Can you work these out from the drawing? Everything is in mm from the part's minimum corner. Round coordinates to 2 decimals unless told otherwise and drop trailing zeros. Loops run counter-clockwise (first coordinate to the right, second up) from the corner with the lowest first, then second, coordinate; pieces in that order, holes last. Notation, with made-up numbers: M -37.75,21.5 L 21.25,21.5 A18 cw 21.25,41.5 Z; hole C 75,23.5 d7. An arc over 180 degrees is marked long. Use a Markdown table: item, result.
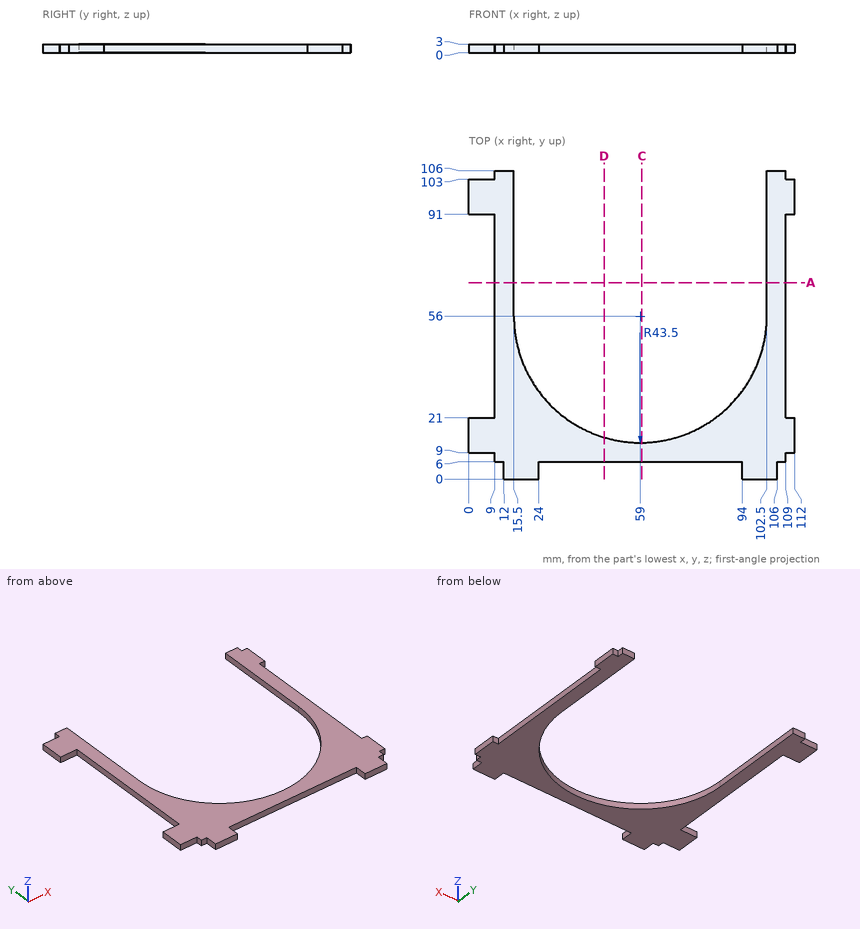
1. Imagine slicing it at D-D, the plane x = 46.5. Write out the boundary of the cut face in (y, z).
Answer sheet:
| item | result |
|---|---|
| outline | M 6,0 L 14.33,0 L 14.33,3 L 6,3 Z |
2. Imagine slicing it at C-C, the plane x = 59.5. Write out the boundary of the cut face in (y, z).
Answer sheet:
| item | result |
|---|---|
| outline | M 6,0 L 12.5,0 L 12.5,3 L 6,3 Z |
3. I need wall thicknesses on probe 1 along X at (y, z) = (63.5, 2.6); probe 2 along Y at (x, z) = (5, 1.8); probe 3 along X at (y, z) = (5.5, 0.25). Which ranges of each line are inside material? Lowest first, please. Write a range as from..to.
Answer sheet:
| item | result |
|---|---|
| probe 1 | 9..15.5, 102.5..109 |
| probe 2 | 9..21, 91..103 |
| probe 3 | 12..24, 94..106 |
4. Imagine slicing it at A-A, the plane y = 67.5. Write out the boundary of the cut face in (x, z).
Answer sheet:
| item | result |
|---|---|
| outline | M 9,0 L 15.5,0 L 15.5,3 L 9,3 Z; M 102.5,0 L 109,0 L 109,3 L 102.5,3 Z |
5. For pin 1 Ø0.9 at (y, z) = (2.5, 1.5) entering from +X; pin 2 Ø0.9 at (x, z) = (107, 2) entering from -Y; pin 3 Ø0.9 at (y, z) = (82.5, 1) entering from -X, each with a flat end and sliding along its axis, tell me the tip position at first contact or that it passes through.
Answer sheet:
| item | result |
|---|---|
| pin 1 | x = 106 |
| pin 2 | y = 6 |
| pin 3 | x = 9 |
